from build123d import *

# Parameters (mm, degrees)
SKETCH1_W               = 44.958
SKETCH1_H               = 304.8
BOSS_EXTRUDE1_DEPTH     = 3.175
BOSS_EXTRUDE2_DEPTH     = 3.175
SKETCH3_W               = 123.825
SKETCH3_H               = 6.35
BOSS_EXTRUDE3_DEPTH     = 41.783
SKETCH8_W               = 3.175
SKETCH8_H               = 213.451350416
CUT_EXTRUDE4_DEPTH      = 1
CUT_EXTRUDE4_DEPTH_BACK = 131.175
SKETCH6_W               = 3.175
SKETCH6_H               = 12.7
CUT_EXTRUDE5_DEPTH      = 3.175
SKETCH4_3_W             = 6.35
SKETCH4_3_H             = 15.875
SKETCH4_3_H_2           = 5.588
SKETCH4_3_H_3           = 7.112
CUT_EXTRUDE6_DEPTH      = 6.35


with BuildPart() as part:
    # Sketch1 → Boss-Extrude1 (new body)
    with BuildSketch(Plane.XY):
        with Locations((-6.477, 3.048)):
            Rectangle(SKETCH1_W, SKETCH1_H)
        with BuildLine():
            Line((-3.302, 133.858), (-3.302, -143.002))
            Line((-3.302, -143.002), (3.302, -143.002))
            Line((3.302, -143.002), (3.302, 143.002))
            Line((3.302, 143.002), (-16.256, 143.002))
            Line((-16.256, 143.002), (-16.256, 136.398))
            Line((-16.256, 136.398), (-5.842, 136.398))
            ThreePointArc((-5.842, 136.398), (-4.045948776, 135.654051224), (-3.302, 133.858))
        make_face(mode=Mode.SUBTRACT)
    extrude(amount=BOSS_EXTRUDE1_DEPTH)

    # Sketch2 → Boss-Extrude2 (add)
    with BuildSketch(Plane(origin=(16.002, 0, 0), x_dir=(0, 0, -1), z_dir=(1, 0, 0))):
        Polygon((123.825, -47.752), (-3.175, -47.752), (-3.175, -149.352), (123.825, -149.352), (123.825, -136.652), (127, -136.652), (127, -119.718666667), (123.825, -119.718666667), (123.825, -107.018666667), (127, -107.018666667), (127, -90.085333333), (123.825, -90.085333333), (123.825, -77.385333333), (127, -77.385333333), (127, -60.452), (123.825, -60.452), align=None)
        with BuildLine():
            ThreePointArc((11.9, -106.092), (10.4, -107.592), (8.9, -106.092))
            Line((8.9, -106.092), (8.9, -101.012))
            ThreePointArc((8.9, -101.012), (10.4, -99.512), (11.9, -101.012))
            Line((11.9, -101.012), (11.9, -106.092))
        make_face(mode=Mode.SUBTRACT)
        with BuildLine():
            ThreePointArc((60.9, -106.092), (59.4, -107.592), (57.9, -106.092))
            Line((57.9, -106.092), (57.9, -101.012))
            ThreePointArc((57.9, -101.012), (59.4, -99.512), (60.9, -101.012))
            Line((60.9, -101.012), (60.9, -106.092))
        make_face(mode=Mode.SUBTRACT)
        with BuildLine():
            Line((8.9, -96.092), (8.9, -91.012))
            ThreePointArc((8.9, -91.012), (10.4, -89.512), (11.9, -91.012))
            Line((11.9, -91.012), (11.9, -96.092))
            ThreePointArc((11.9, -96.092), (10.4, -97.592), (8.9, -96.092))
        make_face(mode=Mode.SUBTRACT)
        with BuildLine():
            ThreePointArc((36.4, -101.092), (25.4, -112.092), (14.4, -101.092))
            Line((14.4, -101.092), (14.4, -96.012))
            ThreePointArc((14.4, -96.012), (25.4, -85.012), (36.4, -96.012))
            Line((36.4, -96.012), (36.4, -101.092))
        make_face(mode=Mode.SUBTRACT)
        with BuildLine():
            ThreePointArc((57.9, -91.012), (59.4, -89.512), (60.9, -91.012))
            Line((60.9, -91.012), (60.9, -96.092))
            ThreePointArc((60.9, -96.092), (59.4, -97.592), (57.9, -96.092))
            Line((57.9, -96.092), (57.9, -91.012))
        make_face(mode=Mode.SUBTRACT)
    extrude(amount=-BOSS_EXTRUDE2_DEPTH)

    # Sketch3 → Boss-Extrude3 (add)
    with BuildSketch(Plane.ZY.offset(-12.827)):
        with Locations((-61.9125, -146.177)):
            Rectangle(SKETCH3_W, SKETCH3_H)
    extrude(amount=BOSS_EXTRUDE3_DEPTH)

    # Sketch8 → Cut-Extrude4 (cut, two sides)
    with BuildSketch(Plane.XY.offset(3.175)) as cut_extrude4_sk:
        Polygon((-28.956, -149.352), (12.827, -149.352), (12.827, -47.752), (12.827, 155.448), (-28.956, 155.448), align=None)
        with BuildLine():
            Line((-16.256, 136.398), (-16.256, 143.002))
            Line((-16.256, 143.002), (3.302, 143.002))
            Line((3.302, 143.002), (3.302, -143.002))
            Line((3.302, -143.002), (-3.302, -143.002))
            Line((-3.302, -143.002), (-3.302, 133.858))
            ThreePointArc((-3.302, 133.858), (-4.045948776, 135.654051224), (-5.842, 136.398))
            Line((-5.842, 136.398), (-16.256, 136.398))
        make_face(mode=Mode.SUBTRACT)
        Polygon((-54.223542679, -149.352), (-28.956, -149.352), (-28.956, 155.448), (12.827, 155.448), (12.827, 165.699350416), (-54.223542679, 165.699350416), align=None)
        with Locations((14.4145, 58.973675208)):
            Rectangle(SKETCH8_W, SKETCH8_H)
    extrude(amount=CUT_EXTRUDE4_DEPTH, mode=Mode.SUBTRACT)
    extrude(cut_extrude4_sk.sketch, amount=-CUT_EXTRUDE4_DEPTH_BACK, mode=Mode.SUBTRACT)

    # Sketch6 → Cut-Extrude5 (cut)
    with BuildSketch(Plane.XY.offset(3.175)):
        with Locations((14.4145, -54.102)):
            Rectangle(SKETCH6_W, SKETCH6_H)
        with Locations((14.4145, -83.735333333)):
            Rectangle(SKETCH6_W, SKETCH6_H)
        with Locations((14.4145, -113.368666667)):
            Rectangle(SKETCH6_W, SKETCH6_H)
        with Locations((14.4145, -143.002)):
            Rectangle(SKETCH6_W, SKETCH6_H)
    extrude(amount=-CUT_EXTRUDE5_DEPTH, mode=Mode.SUBTRACT)

    # Sketch4<3> → Cut-Extrude6 (cut)
    with BuildSketch(Plane.XZ.offset(149.352)):
        with Locations((12.827, -103.1875)):
            Rectangle(SKETCH4_3_W, SKETCH4_3_H)
        with Locations((12.827, -74.6125)):
            Rectangle(SKETCH4_3_W, SKETCH4_3_H)
        with Locations((12.827, -46.0375)):
            Rectangle(SKETCH4_3_W, SKETCH4_3_H)
        with Locations((12.827, -17.4625)):
            Rectangle(SKETCH4_3_W, SKETCH4_3_H)
        with Locations((12.827, 0.381)):
            Rectangle(SKETCH4_3_W, SKETCH4_3_H_2)
        with Locations((12.827, -5.969)):
            Rectangle(SKETCH4_3_W, SKETCH4_3_H_3)
    extrude(amount=-CUT_EXTRUDE6_DEPTH, mode=Mode.SUBTRACT)


solid = part.part
For this review, take the finished solid that the model builds, in its own axes (mm). A direction names the side the tool comes from. Round coordinates to 2 decimals unless told otherwise and drop trailing zeros. Loops run counter-clockwise (first coordinate to the right, second up) from the corner with the lowest first, then second, coordinate; pieces in that order, holes last. Notation, with made-up numbers: (-7, 89.25) - (51, 89.25) arc R11 ccw to (51, 109.25) - close; hole circle Ø3 at (-26, -32). An arc over 180 degrees is marked (long way). One line per item, written item: value. Start each with the question number.
Item 1: Take a section at D-D (z = -59.4). Give the boundary of the cut face in (x, y), plus the area to 3 significant figures.
Item 2: Clearance check with flat-ended pins moving along their axes: pin 1 Ø1 at (x, z) = (15.5, -39) entering from -Y; pin 2 Ø1 at (x, y) = (15, -146) entering from +Z; pin 3 Ø1 at (x, z) = (15, -125.5) entering from +Y. State where each tip first meets the part, or that it passes through.
Item 3: The part is to be moulded in two halves that separate along Z. For faces 4 (the cylindrical face through (14.44, -107.59, -10.43)), 5 (the flat face through (14, -60.452, 2)), 6 (the flat face through (14, -69, -127)), say which applies: +Z half, -Z half, draft (parallel to the pull), parting line (faces both ways), or undercut.
Item 4: For faces 1 (the flat face through (14, -146, -111.125)), 2 (the flat face through (14, -113, -123.825)), 3 (the cylindrical face through (14.437, -99.512, -59.367)), list the 3-axis set-ups (+Z, -Z, +X, -X, +Y, -Y) from which the entire face can be reached by the end or side of a thin tool; tool diameter is ignored.
Item 5: Take a section at C-C (x = 14.65). State how many separate pieces and enclosed holes the cut face has, plus the area to 3 significant figures.
Item 6: Take a section at A-A (z = -10.4). Give the boundary of the cut face in (x, y), plus the area to 3 significant figures.
Item 7: For L1, parallel to Z at x = 15.8, y = -103.5 (3 decimals); L2, parallel to Z at x = 14.4, y = -145 (3 decimals); L3, parallel to Y at x = 14.7, z = -6, list the stretches that pass through material, from the lowest coordinate up.
Item 8: Take a section at B-B (y = -103.5). Give the boundary of the cut face in (x, z) (3 decimals).
Answer below:
1. outline: (12.83, -149.35) - (16, -149.35) - (16, -107.59) - (12.83, -107.59) - close; (12.83, -99.51) - (16, -99.51) - (16, -97.59) - (12.83, -97.59) - close; (12.83, -89.51) - (16, -89.51) - (16, -47.75) - (12.83, -47.75) - close
1. area: 271 mm2
2. pin 1: stops at y = -143
2. pin 2: stops at z = -25.4
2. pin 3: stops at y = -60.45
3. face 4: undercut
3. face 5: draft
3. face 6: -Z half
4. face 1: +X, -X, -Y
4. face 2: -Z, +X, -X
4. face 3: +X, -X
5. separate pieces: 1
5. enclosed holes: 5
5. area: 11,900 mm2
6. outline: (12.83, -143) - (16, -143) - (16, -107.59) - (12.83, -107.59) - close; (12.83, -99.51) - (16, -99.51) - (16, -97.59) - (12.83, -97.59) - close; (12.83, -89.51) - (16, -89.51) - (16, -47.75) - (12.83, -47.75) - close
6. area: 251 mm2
7. L1: z = -127 to -60.9, -57.9 to -36.133, -14.667 to -11.9, -8.9 to 3.175
7. L2: z = -123.825 to -111.125, -95.25 to -82.55, -66.675 to -53.975, -38.1 to -25.4
7. L3: y = -143 to -47.75
8. outline: (12.827, -127) - (16.002, -127) - (16.002, -60.9) - (12.827, -60.9) - close; (12.827, -57.9) - (16.002, -57.9) - (16.002, -36.133) - (12.827, -36.133) - close; (12.827, -14.667) - (16.002, -14.667) - (16.002, -11.9) - (12.827, -11.9) - close; (12.827, -8.9) - (16.002, -8.9) - (16.002, 3.175) - (12.827, 3.175) - close
